For this review, take the finished solid that the model builds, in its own axes (mm). A direction names the side the tool comes from. Coordinates: 2 decimals unless noted, no trailing zeros. Loops run counter-clockwise (first coordinate to the right, second up) from the corner with the lowest first, then second, coordinate; pieces in that order, holes last. Notation, with made-up numbers: (31, 83.5) - (43, 83.5) arc R28 cw to (43, 108.5) - close; hole circle Ø7 at (-28.75, 20). An arc over 180 degrees is marked (long way). One line per item, written item: value. Start each with the question number.
1. Take a section at A-A, the plane z = 0. State the section outline as (x, y) points (3 decimals), and give its area (3 significant figures).
2. Insertion check: pin 1 (1 mm diameter, centred on y = 4.5, z = -18, fed in from +X); pin 2 (1.7 mm diameter, centred on x = 0.5, y = 4.5, fed in from +Z); pin 3 (2 mm diameter, centred on y = 1, z = -13.5, fed in from +X); pin 4 (9.5 mm diameter, centred on x = -6.5, z = 3, fed in from -Y). Each pin has a flat end and moves straight along its axis. Give the tip position at first contact, or say it passes through.
3. For faces 4 (the face through (0, 5, -3)), 5 (the face through (0, 3, -4)), 6 (the face through (172.395, 3.131, 0.44)), list the 3-axis set-ups (+Z, -Z, +X, -X, +Y, -Y) from which the entire face can be reached by the end or side of a thin tool; tool diameter is ignored.
4. Take a section at C-C, the plane x = 136. State the section outline as (y, z) points.
5. To check wall thickness, follow line 1 (X direction, y = 0.5, z = -7.5); line 2 (X direction, y = 5.5, z = 0) (3 decimals); line 3 (Z direction, x = 152.4, y = 2.5) (3 decimals). State the ranges of each line that lie inside material, in increasing order. Write a range as from..to.
6. The part is to be moulded in two halves that separate along Z. For faces 1 (the face through (70, 0, 0)), 2 (the face through (-29.993, 3.131, -0.66)), 3 (the face through (0, 5, 4)), say which applies: released by +Z, released by -Z, zero draft, split by the parting line, or undercut.
7. Take a section at D-D, the plane z = 24.5. State the section outline as (x, y) points.
8. Take a section at B-B, the plane y = 5. Count the separate pieces of the cut face and the enclosed holes in it, and give its area (3 significant figures).
```python
from build123d import *

# Parameters (mm, degrees)
SKETCH2_R             = 20
BOSS_EXTRUDE1_DEPTH   = 6.35
SKETCH11_R            = 3.175
CUT_EXTRUDE1_DEPTH    = 10
CUT_EXTRUDE2_START    = -6.35
SKETCH12_R            = 16
CUT_EXTRUDE2_DEPTH    = 3
SKETCH13_R            = 1.95
CUT_EXTRUDE3_DEPTH    = 176.022805657
F_3_0MM_DOWEL_HOLE1_D = 3
CIRPATTERN1_COUNT     = 4


with BuildPart() as part:
    # Sketch2 → Boss-Extrude1 (new body)
    # profile 1 of 3: a face of its own
    with BuildSketch(Plane(origin=(0, 0, 0), x_dir=(1, 0, 0), z_dir=(0, 1, 0))):
        with BuildLine():
            Line((152.4, 20), (3.920129505, 29.742773655))
            ThreePointArc((3.920129505, 29.742773655), (22.556638548, 19.778727397), (30, 0))
            ThreePointArc((30, 0), (22.556638548, -19.778727397), (3.920129505, -29.742773655))
            Line((3.920129505, -29.742773655), (152.4, -20))
            ThreePointArc((152.4, -20), (132.4, 0), (152.4, 20))
        make_face()
    # profile 2 of 3: a face of its own
    with BuildSketch(Plane(origin=(0, 0, 0), x_dir=(1, 0, 0), z_dir=(0, 1, 0))):
        with BuildLine():
            Line((3.920129505, 29.742773655), (0, 30))
            ThreePointArc((0, 30), (-30, 0), (0, -30))
            Line((0, -30), (3.920129505, -29.742773655))
            ThreePointArc((3.920129505, -29.742773655), (22.556638548, -19.778727397), (30, 0))
            ThreePointArc((30, 0), (22.556638548, 19.778727397), (3.920129505, 29.742773655))
        make_face()
        with BuildLine():
            ThreePointArc((2.645751311, 3), (0, -4), (-2.645751311, 3))
            Line((-2.645751311, 3), (2.645751311, 3))
        make_face(mode=Mode.SUBTRACT)
    # profile 3 of 3: a face of its own
    with BuildSketch(Plane(origin=(0, 0, 0), x_dir=(1, 0, 0), z_dir=(0, 1, 0))):
        with Locations((152.4, 0)):
            Circle(SKETCH2_R)
    extrude(amount=BOSS_EXTRUDE1_DEPTH)

    # Sketch11 → Cut-Extrude1 (cut)
    with BuildSketch(Plane(origin=(0, 6.35, 0), x_dir=(1, 0, 0), z_dir=(0, 1, 0))):
        with Locations(Location((152.4, 0, 0), (0, 0, 270))):
            Circle(SKETCH11_R)
    extrude(amount=-CUT_EXTRUDE1_DEPTH, mode=Mode.SUBTRACT)

    # Sketch12 → Cut-Extrude2 (cut)
    with BuildSketch(Plane(origin=(0, 6.35, 0), x_dir=(1, 0, 0), z_dir=(0, 1, 0)).offset(CUT_EXTRUDE2_START)):
        with Locations(Location((0, 0, 0), (0, 0, 270))):
            Circle(SKETCH12_R)
    extrude(amount=CUT_EXTRUDE2_DEPTH, mode=Mode.SUBTRACT)

    # Sketch13 → Cut-Extrude3 (cut, through all)
    with BuildSketch(Plane(origin=(0, 3, 0), x_dir=(-1, 0, 0), z_dir=(0, -1, 0))):
        with Locations(Location((-8.485281374, 8.485281374, 0), (0, 0, 90))):
            Circle(SKETCH13_R)
        with Locations(Location((8.485281374, 8.485281374, 0), (0, 0, 90))):
            Circle(SKETCH13_R)
        with Locations(Location((8.485281374, -8.485281374, 0), (0, 0, 90))):
            Circle(SKETCH13_R)
        with Locations(Location((-8.485281374, -8.485281374, 0), (0, 0, 90))):
            Circle(SKETCH13_R)
    extrude(amount=-CUT_EXTRUDE3_DEPTH, mode=Mode.SUBTRACT)

    # Ø3.0mm Dowel Hole1 (through all)
    with Locations(Plane(origin=(0, 0, 0), x_dir=(-1, 0, 0), z_dir=(0, -1, 0))):
        with Locations((-160.885281374, -8.485281374)):
            f_3_0mm_dowel_hole1 = Hole(F_3_0MM_DOWEL_HOLE1_D / 2)

    # CirPattern1: Ø3.0mm Dowel Hole1 ×4 about axis
    cirpattern1_axis = Axis((152.4, 0, 0), (0, 1, 0))
    for i in range(1, CIRPATTERN1_COUNT):
        add(f_3_0mm_dowel_hole1.rotate(cirpattern1_axis, i * 360 / CIRPATTERN1_COUNT), mode=Mode.SUBTRACT)


solid = part.part
```
Solutions:
1. outline: (-30, 0) - (-16, 0) - (-16, 3) - (-4, 3) - (-4, 6.35) - (-30, 6.35) - close; (4, 3) - (16, 3) - (16, 0) - (149.225, 0) - (149.225, 6.35) - (4, 6.35) - close; (155.575, 0) - (172.4, 0) - (172.4, 6.35) - (155.575, 6.35) - close
1. area: 1,120 mm2
2. pin 1: x = 162.08
2. pin 2: z = 30
2. pin 3: x = 168.01
2. pin 4: y = 3
3. face 4: +Y, -Y
3. face 5: -Y
3. face 6: +X, +Y, -Y
4. outline: (0, -21.08) - (6.35, -21.08) - (6.35, 21.08) - (0, 21.08) - close
5. line 1: -29.05..-14.13, 14.13..142.78, 145.05..159.75, 162.02..170.94
5. line 2: -30..-4, 4..149.225, 155.575..172.4
5. line 3: -20..-3.175, 3.175..20
6. face 1: zero draft
6. face 2: split by the parting line
6. face 3: undercut
7. outline: (-17.31, 0) - (83.82, 0) - (83.82, 6.35) - (-17.31, 6.35) - close
8. separate pieces: 1
8. enclosed holes: 10
8. area: 9,510 mm2
